Verification items for the finished model (mm, model axes). A direction names the side the tool comes from. Round coordinates to 2 decimals unless told otherwise and drop trailing zeros. Loops run counter-clockwise (first coordinate to the right, second up) from the corner with the lowest first, then second, coordinate; pieces in that order, holes last. Notation, with made-up numbers: (37, -32.75) -> (55, -32.75) arc R4 ccw to (55, -28.75) -> close; hole circle Ø11 at (-16, 39). An arc over 180 degrees is marked (long way). Use a Markdown table: item, result. Add a question column.
```python
from build123d import *

# Parameters (mm, degrees)
SKETCH2_R                 = 5
BOSS_EXTRUDE2_DEPTH       = 2
SKETCH3_R                 = 0.8
CUT_EXTRUDE1_DEPTH        = 2
SKETCH4_R                 = 0.8
CUT_EXTRUDE2_DEPTH        = 2
CHAMFER1_SIZE             = 2
CIRPATTERN3_COUNT         = 8
F_2_5MM_DOWEL_HOLE1_D     = 2.5
F_2_5MM_DOWEL_HOLE1_DEPTH = 10
F_2_5MM_DOWEL_HOLE1_TIP   = 0.751075774


with BuildPart() as part:
    # Sketch2 → Boss-Extrude2 (new body)
    with BuildSketch(Plane(origin=(0, 0, 0), x_dir=(1, 0, 0), z_dir=(0, 1, 0))):
        with BuildLine():
            Line((-7, 21.800048896), (-7, 28.000048896))
            Line((-7, 28.000048896), (-11.598, 28.000048896))
            Line((-11.598, 28.000048896), (-14.84927698, 24.748771917))
            Line((-14.84927698, 24.748771917), (-10.465214937, 20.364709873))
            ThreePointArc((-10.465214937, 20.364709873), (-14.786262044, 14.786262044), (-20.364709873, 10.465214937))
            Line((-20.364709873, 10.465214937), (-24.748771917, 14.84927698))
            Line((-24.748771917, 14.84927698), (-28.000048896, 11.598))
            Line((-28.000048896, 11.598), (-28.000048896, 7))
            Line((-28.000048896, 7), (-21.800048896, 7))
            ThreePointArc((-21.800048896, 7), (-20.91093232, 0), (-21.800048896, -7))
            Line((-21.800048896, -7), (-28.000048896, -7))
            Line((-28.000048896, -7), (-28.000048896, -11.598))
            Line((-28.000048896, -11.598), (-24.748771917, -14.84927698))
            Line((-24.748771917, -14.84927698), (-20.364709873, -10.465214937))
            ThreePointArc((-20.364709873, -10.465214937), (-14.786262044, -14.786262044), (-10.465214937, -20.364709873))
            Line((-10.465214937, -20.364709873), (-14.84927698, -24.748771917))
            Line((-14.84927698, -24.748771917), (-11.598, -28.000048896))
            Line((-11.598, -28.000048896), (-7, -28.000048896))
            Line((-7, -28.000048896), (-7, -21.800048896))
            ThreePointArc((-7, -21.800048896), (0, -20.91093232), (7, -21.800048896))
            Line((7, -21.800048896), (7, -28.000048896))
            Line((7, -28.000048896), (11.598, -28.000048896))
            Line((11.598, -28.000048896), (14.84927698, -24.748771917))
            Line((14.84927698, -24.748771917), (10.465214937, -20.364709873))
            ThreePointArc((10.465214937, -20.364709873), (14.786262044, -14.786262044), (20.364709873, -10.465214937))
            Line((20.364709873, -10.465214937), (24.748771917, -14.84927698))
            Line((24.748771917, -14.84927698), (28.000048896, -11.598))
            Line((28.000048896, -11.598), (28.000048896, -7))
            Line((28.000048896, -7), (21.800048896, -7))
            ThreePointArc((21.800048896, -7), (20.91093232, 0), (21.800048896, 7))
            Line((21.800048896, 7), (28.000048896, 7))
            Line((28.000048896, 7), (28.000048896, 11.598))
            Line((28.000048896, 11.598), (24.748771917, 14.84927698))
            Line((24.748771917, 14.84927698), (20.364709873, 10.465214937))
            ThreePointArc((20.364709873, 10.465214937), (14.786262044, 14.786262044), (10.465214937, 20.364709873))
            Line((10.465214937, 20.364709873), (14.84927698, 24.748771917))
            Line((14.84927698, 24.748771917), (11.598, 28.000048896))
            Line((11.598, 28.000048896), (7, 28.000048896))
            Line((7, 28.000048896), (7, 21.800048896))
            ThreePointArc((7, 21.800048896), (0, 20.91093232), (-7, 21.800048896))
        make_face()
        Circle(SKETCH2_R, mode=Mode.SUBTRACT)
    extrude(amount=BOSS_EXTRUDE2_DEPTH)

    # Sketch3 → Cut-Extrude1 (cut)
    with BuildSketch(Plane.ZY.offset(-7)):
        with Locations((-26.000048896, 0)):
            Circle(SKETCH3_R)
    cut_extrude1 = extrude(amount=-CUT_EXTRUDE1_DEPTH, mode=Mode.SUBTRACT)

    # Sketch4 → Cut-Extrude2 (cut)
    with BuildSketch(Plane(origin=(-7, 0, 0), x_dir=(0, 0, -1), z_dir=(1, 0, 0))):
        with Locations((26.000048896, 0)):
            Circle(SKETCH4_R)
    cut_extrude2 = extrude(amount=-CUT_EXTRUDE2_DEPTH, mode=Mode.SUBTRACT)

    # Chamfer1
    chamfer1_edges = [part.edges().sort_by_distance(p)[0] for p in [
        (-11.598, 1, -28.000048896),
        (11.598, 1, -28.000048896),
        (28.000048896, 1, -11.598),
        (28.000048896, 1, 11.598),
        (11.598, 1, 28.000048896),
        (-11.598, 1, 28.000048896),
        (-28.000048896, 1, 11.598),
        (-28.000048896, 1, -11.598),
    ]]
    chamfer(chamfer1_edges, length=CHAMFER1_SIZE)

    # CirPattern3: Cut-Extrude1, Cut-Extrude2 ×8 about axis
    cirpattern3_axis = Axis((0, 0, 0), (0, 1, 0))
    for i in range(1, CIRPATTERN3_COUNT):
        add(cut_extrude1.rotate(cirpattern3_axis, i * 360 / CIRPATTERN3_COUNT), mode=Mode.SUBTRACT)
        add(cut_extrude2.rotate(cirpattern3_axis, i * 360 / CIRPATTERN3_COUNT), mode=Mode.SUBTRACT)

    # Ø2.5mm Dowel Hole1
    with Locations(Plane(origin=(0, 2, 0), x_dir=(1, 0, 0), z_dir=(0, 1, 0))):
        with Locations((0, 12), (10.392304845, -6), (-10.392304845, -6), (0, 0)):
            Hole(F_2_5MM_DOWEL_HOLE1_D / 2, depth=F_2_5MM_DOWEL_HOLE1_DEPTH)
            with Locations((0, 0, -(F_2_5MM_DOWEL_HOLE1_DEPTH + F_2_5MM_DOWEL_HOLE1_TIP / 2))):  # 118° drill point
                Cone(0, F_2_5MM_DOWEL_HOLE1_D / 2, F_2_5MM_DOWEL_HOLE1_TIP, mode=Mode.SUBTRACT)


solid = part.part
```
1) Sectioned sample at A-A on x = 0. Enter the section's corners in (y, z).
2) Sectioned sample at C-C on y = 1.2. State how many separate pieces and enclosed holes the cut face has, then the cut area to 3 significant figures.
3) Sectioned sample at B-B on z = 3.5. Enter the section's corners in (x, y), then the cut area to 3 significant figures.
4) Sectioned sample at D-D on z = 18. Enter the section's corners in (x, y), then the cut area to 3 significant figures.
5) Thickness scan on line 1 (Z direction, x = 0, y = 1.25); line 2 (X direction, y = 1.1, z = 0); line 3 (X direction, y = 1.35, z = 6). Record the ranges inside material, lowest first.
6) Release check for a two-part mould opening along X. For faces 4 (the face through (13.9, 1, -25.7)), 5 (the face through (25, 1, 7)), 6 (the face through (-22.5, 1, -12.6)), 7 (the face through (-20.91, 0.99, -0.1)) record: released by +X, released by -X, zero draft, split by the parting line, or undercut.
7) Access from +Z, -Z, +X, -X, +Y, -Y to the whole of each face (thin tool, end or side, straight path). Record for faces 1 (the face through (22.5, 1, 12.6)), 2 (the face through (-26, 0.8, 8)), 3 (the face through (-14.856, 0.986, 14.716)).
8) Go/stop test with flat-tipped pins: pin 1 (0.6 mm diameter, centred on x = -25.5, y = 0.5, fed in from -Z); pin 2 (1.5 mm diameter, centred on x = 5.5, z = 20, fed in from -Y); pin 3 (0.6 mm diameter, centred on y = 0.5, z = -25.5, fed in from -X); pin 4 (1 mm diameter, centred on x = -25.5, y = 0.5, fed in from -Z). Record where each tip stops, or that it passes through.
Geometry results:
| question | item | result |
|---|---|---|
| 1 | outline | (0, -20.91) -> (2, -20.91) -> (2, -13.25) -> (0, -13.25) -> close; (0, -10.75) -> (2, -10.75) -> (2, -5) -> (0, -5) -> close; (0, 5) -> (2, 5) -> (2, 20.91) -> (0, 20.91) -> close |
| 2 | separate pieces | 1 |
| 2 | enclosed holes | 4 |
| 2 | area | 1,730 mm^2 |
| 3 | outline | (-21.13, 0) -> (-3.57, 0) -> (-3.57, 2) -> (-21.13, 2) -> close; (3.57, 0) -> (21.13, 0) -> (21.13, 2) -> (3.57, 2) -> close |
| 3 | area | 70.2 mm^2 |
| 4 | outline | (-12.03, 0) -> (12.03, 0) -> (12.03, 2) -> (-12.03, 2) -> close |
| 4 | area | 48.1 mm^2 |
| 5 | line 1 | -20.91 to -13.25, -10.75 to -5, 5 to 20.91 |
| 5 | line 2 | -20.91 to -5, 5 to 20.91 |
| 5 | line 3 | -21.56 to -11.64, -9.14 to 9.14, 11.64 to 21.56 |
| 6 | face 4 | released by +X |
| 6 | face 5 | zero draft |
| 6 | face 6 | undercut |
| 6 | face 7 | released by -X |
| 7 | face 1 | +Z, +Y, -Y |
| 7 | face 2 | -Y |
| 7 | face 3 | +Y, -Y |
| 8 | pin 1 | z = -14.4 |
| 8 | pin 2 | y = 0 |
| 8 | pin 3 | x = -14.4 |
| 8 | pin 4 | z = -14.6 |
